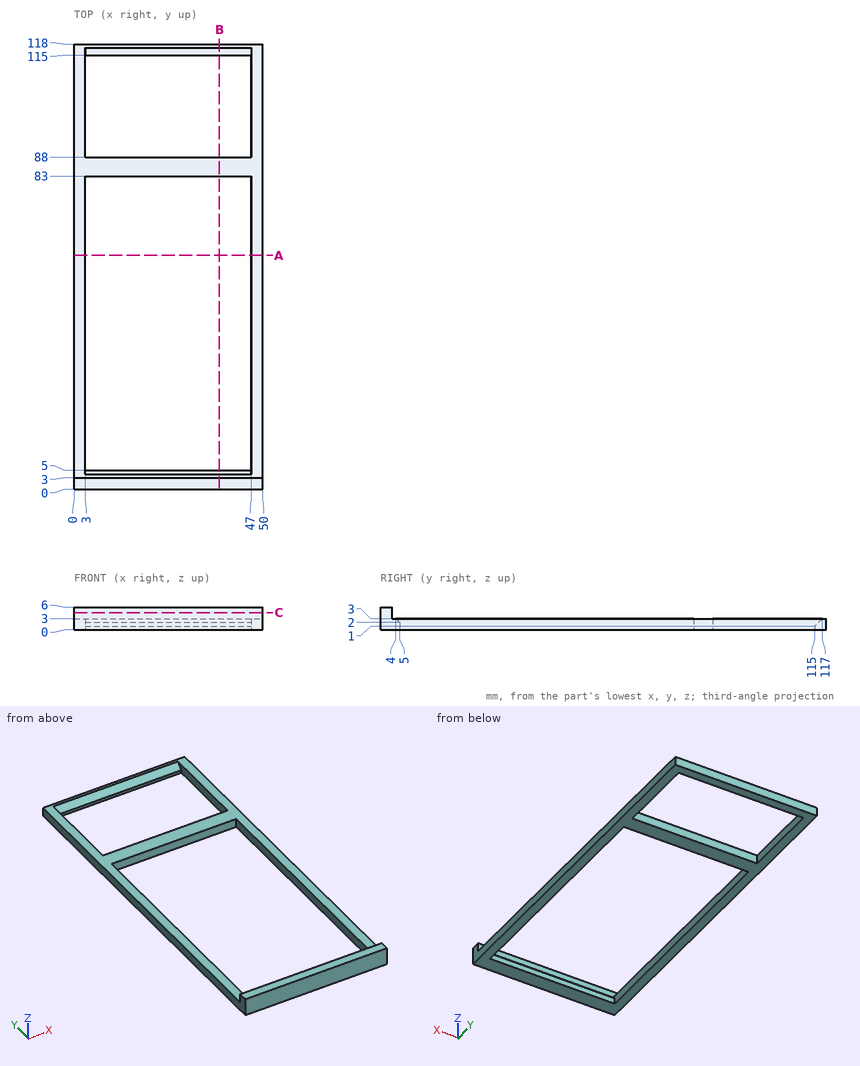
Geometry: see drawing. Coordinates: mm, zero at the bounding-box minimum. Coordinates: 2 decimals unless noted, no trailing zeros. Order: outer loops, then holes, each group sorted by start corner. A loop starts at its lowest first (then second) coordinate and runs counter-clockwise, first axis right, second up. Notation, with made-up numbers: M -34.75,-29.75 L -28.75,-29.75 A29 cw -28.75,-7.75 Z; hole C 79,67.5 d9. An arc over 180 degrees is marked long. Write item = value, one per line. Start each with the question number.
(1) First-contact query: P1, Ø3, axis at x = 33.5, y = 85.5, coming from the +Z side; P2, Ø8, axis at x = 33, y = 12, coming from the +Z side. Flat tips, straight axial feed; report the tip coordinate or a pass-through.
(2) Line query: line 1 along Y through (x, z) = (5.5, 0.4); line 2 along X through (y, z) = (64, 0.8); line 3 along Y through (x, z) = (13, 4.95). Output: solid intervals per line, ascending. Write a range as [from, to].
(3) Section A-A on y = 62. Output: boundary loops of the cut face in (x, z), and give its area (3 significant figures).
(4) Section B-B on x = 38.5. Output: boundary loops of the cut face in (y, z), and give its area (3 significant figures).
(5) Section C-C on z = 4.6. Output: boundary loops of the cut face in (x, y).
Result set:
q1.P1 = 3
q1.P2 = through
q2.line_1 = [0, 5], [83, 88], [115, 118]
q2.line_2 = [0, 3], [47, 50]
q2.line_3 = [0, 3]
q3.outline = M 0,0 L 3,0 L 3,3 L 0,3 Z; M 47,0 L 50,0 L 50,3 L 47,3 Z
q3.area = 18.0 mm²
q4.outline = M 0,0 L 5,0 L 5,2 L 4,3 L 3,3 L 3,6 L 0,6 Z; M 83,0 L 88,0 L 88,3 L 83,3 Z; M 115,0 L 118,0 L 118,3 L 117,3 L 115,1 Z
q4.area = 45.5 mm²
q5.outline = M 0,0 L 50,0 L 50,3 L 0,3 Z
